```python
from build123d import *

# Parameters (mm, degrees)
SKETCH_1_W          = 200
SKETCH_1_H          = 200
EXTRUDE_1_DEPTH     = 10
SKETCH_2_W          = 15.7
SKETCH_2_H          = 95
EXTRUDE_2_DEPTH     = 130
SKETCH_3_R          = 1.75
CUT_EXTRUDE_1_DEPTH = 259.650343128
SKETCH_4_R          = 29
CUT_EXTRUDE_2_DEPTH = 500
SKETCH_5_W          = 51.576818731
SKETCH_5_H          = 51.835019378
SKETCH_5_W_2        = 50.790053699
SKETCH_5_H_2        = 44.901224563
CUT_EXTRUDE_3_DEPTH = 259.650343128
SKETCH_6_R          = 2.5
CUT_EXTRUDE_4_DEPTH = 259.650343128
FILLET_1_R          = 25
SKETCH_7_R          = 2
CUT_EXTRUDE_5_DEPTH = 193.093727123


with BuildPart() as part:
    # 草图1 → 凸台-拉伸1 (new body)
    with BuildSketch(Plane.XY):
        Rectangle(SKETCH_1_W, SKETCH_1_H)
    extrude(amount=EXTRUDE_1_DEPTH)

    # 草图2 → 凸台-拉伸2 (add)
    with BuildSketch(Plane(origin=(0, 0, 0), x_dir=(-1, 0, 0), z_dir=(0, 0, -1))):
        with Locations((-92.15, 0)):
            Rectangle(SKETCH_2_W, SKETCH_2_H)
        with Locations((92.15, 0)):
            Rectangle(SKETCH_2_W, SKETCH_2_H)
    extrude(amount=EXTRUDE_2_DEPTH)

    # 草图3 → 切除-拉伸1 (cut, through all)
    with BuildSketch(Plane.ZY.offset(100)):
        with Locations(Location((-81.75, -42.5, 0), (0, 0, 270))):
            Circle(SKETCH_3_R)
        with Locations(Location((-51.6979618, -30.0520382, 0), (0, 0, 270))):
            Circle(SKETCH_3_R)
        with Locations(Location((-39.25, 0, 0), (0, 0, 270))):
            Circle(SKETCH_3_R)
        with Locations(Location((-81.75, 42.5, 0), (0, 0, 270))):
            Circle(SKETCH_3_R)
        with Locations(Location((-111.8020382, 30.0520382, 0), (0, 0, 270))):
            Circle(SKETCH_3_R)
        with Locations(Location((-111.8020382, -30.0520382, 0), (0, 0, 270))):
            Circle(SKETCH_3_R)
        with Locations(Location((-51.6979618, 30.0520382, 0), (0, 0, 270))):
            Circle(SKETCH_3_R)
        with Locations(Location((-124.25, 0, 0), (0, 0, 270))):
            Circle(SKETCH_3_R)
    extrude(amount=-CUT_EXTRUDE_1_DEPTH, mode=Mode.SUBTRACT)

    # 草图4 → 切除-拉伸2 (cut, symmetric)
    with BuildSketch(Plane.ZY.offset(-84.3)):
        with Locations((-81.75, 0)):
            Circle(SKETCH_4_R)
    extrude(amount=CUT_EXTRUDE_2_DEPTH, both=True, mode=Mode.SUBTRACT)

    # 草图5 → 切除-拉伸3 (cut, through all)
    with BuildSketch(Plane(origin=(100, 0, 0), x_dir=(0, 0, -1), z_dir=(1, 0, 0))):
        with Locations((107.073919085, 0)):
            Rectangle(SKETCH_5_W, SKETCH_5_H)
        with Locations((49.973585145, -0.398574081)):
            Rectangle(SKETCH_5_W_2, SKETCH_5_H_2)
    extrude(amount=-CUT_EXTRUDE_3_DEPTH, mode=Mode.SUBTRACT)

    # 草图6 → 切除-拉伸4 (cut, through all)
    with BuildSketch(Plane.ZY.offset(100)):
        with Locations(Location((-19.063545362, -36.423322267, 0), (0, 0, 270))):
            Circle(SKETCH_6_R)
        with Locations((-19.063545362, 36.423322267)):
            Circle(SKETCH_6_R)
    extrude(amount=-CUT_EXTRUDE_4_DEPTH, mode=Mode.SUBTRACT)

    # 圆角1
    fillet_1_edges = [part.edges().sort_by_distance(p)[0] for p in [
        (100, -100, 5),
        (-100, -100, 5),
        (-100, 100, 5),
        (100, 100, 5),
    ]]
    fillet(fillet_1_edges, radius=FILLET_1_R)

    # 草图7 → 切除-拉伸5 (cut, through all)
    with BuildSketch(Plane(origin=(0, 0, 0), x_dir=(-1, 0, 0), z_dir=(0, 0, -1))):
        with Locations((17.25, 0)):
            Circle(SKETCH_7_R)
        with Locations((8.625, -14.938938215)):
            Circle(SKETCH_7_R)
        with Locations((-8.625, -14.938938215)):
            Circle(SKETCH_7_R)
        with Locations((-17.25, 0)):
            Circle(SKETCH_7_R)
        with Locations((-8.625, 14.938938215)):
            Circle(SKETCH_7_R)
        with Locations((8.625, 14.938938215)):
            Circle(SKETCH_7_R)
    extrude(amount=-CUT_EXTRUDE_5_DEPTH, mode=Mode.SUBTRACT)


solid = part.part
```
Check sheet for the modelled part. Datum: model origin and axes. Units: mm. A direction names the side the tool comes from. Round coordinates to 2 decimals unless told otherwise and drop trailing zeros. Loops run counter-clockwise (first coordinate to the right, second up) from the corner with the lowest first, then second, coordinate; pieces in that order, holes last. Notation, with made-up numbers: M -38.75,54 L -14.75,54 A13 cw -14.75,59 Z; hole C 4.5,12 d4. An arc over 180 degrees is marked long. Answer as a JSON object with one key per item and string values.
1. Gauge pin test, flat ends, axial feed: P1, Ø4.5, axis at x = -89.5, z = -108.5, coming from the +Y side; P2, Ø10, axis at x = 62.5, y = 0, coming from the -Z side; P3, Ø17.5, axis at x = 95.5, y = 5, coming from the -Z side; P4, Ø3, axis at x = -8.62, y = 14.94, coming from the +Z side. Record the tip position at first contact, or that the pin passes through.
Reply:
{"P1": "stops at y = 47.5", "P2": "stops at z = 0", "P3": "stops at z = -24.58", "P4": "passes through"}
2. Section check B-B (y = 71). Record the boundary of the cut face in (x, z).
Reply:
{"outline": "M -100,0 L 100,0 L 100,10 L -100,10 Z"}
3. Section check A-A (z = -90). Record the boundary of the cut face in (x, y), plus the area to 3 significant figures.
Reply:
{"outline": "M -100,-47.5 L -84.3,-47.5 L -84.3,-27.8 L -100,-27.8 Z; M -100,27.8 L -84.3,27.8 L -84.3,47.5 L -100,47.5 Z; M 84.3,-47.5 L 100,-47.5 L 100,-27.8 L 84.3,-27.8 Z; M 84.3,27.8 L 100,27.8 L 100,47.5 L 84.3,47.5 Z", "area": "1,240 mm²"}
4. Access from +Z, -Z, +X, -X, +Y, -Y to the whole of each face (thin tool, end or side, straight path). Record for faces 1 (the cylindrical face through (-92.26, 28.76, -78.02)), 2 (the flat face through (92, -37, -130)), 3 (the flat face through (92, 47.5, -64)), 4 (the flat face through (-84.3, -32, -50)), 5 (the flat face through (-92, -1, -24.579)).
Reply:
{"face 1": "+X, -X", "face 2": "-Z, +X, -X, +Y, -Y", "face 3": "-Z, +X, -X, +Y", "face 4": "-Z, +Y, -Y", "face 5": "-Z, +X, -X"}
5. Mould release check, pull along Y, two halves, no side actions. Record for faces 6 (the flat face through (-100, 0, -24)), 7 (the flat face through (-1, -100, 5)), 8 (the flat face through (92, 25.918, -112)): pulls with the +Y half, pulls with the -Y half, needs draft (parallel to the pull), parting line crosses it, or undercut.
Reply:
{"face 6": "needs draft", "face 7": "pulls with the -Y half", "face 8": "undercut"}
6. Scan lines: line 1 (Y direction, x = 94.25, z = -81.75); line 2 (X direction, y = -32, z = -43); line 3 (Y direction, x = -87.5, z = -97.5). Record each from-to range of solid material in increasing order.
Reply:
{"line 1": "y = -47.5 to -44.25, -40.75 to -29, 29 to 40.75, 44.25 to 47.5", "line 2": "x = -100 to -84.3, 84.3 to 100", "line 3": "y = -47.5 to -25.92, 25.92 to 47.5"}
